The listing builds one solid part. Answer for the finished solid, in the listing's coordinates (mm). Give positions to 0.01 mm unless a question says otherwise; leave off trailing zeros. Order: outer loops, then holes, each group sorted by start corner. A loop starts at its lowest first (then second) coordinate and runs counter-clockwise, first axis right, second up. Notation, with made-up numbers: (76.25, 67.25) -> (105.25, 67.25) arc R34 cw to (105.25, 105.25) -> close; hole circle Ø3 at (32, 82). An arc over 180 degrees is marked (long way). One line per question, with ' | ' between items. Start each with the question number.
```python
from build123d import *

# Parameters (mm, degrees)
SKETCH1_R           = 28.194
BOSS_EXTRUDE1_DEPTH = 343
SKETCH5_R           = 28.194
BOSS_EXTRUDE3_DEPTH = 245
SKETCH7_R           = 3.675
CUT_EXTRUDE1_DEPTH  = 369.4


with BuildPart() as part:
    # Sketch1 → Boss-Extrude1 (new body)
    with BuildSketch(Plane(origin=(0, 0, 0), x_dir=(0, 0, -1), z_dir=(1, 0, 0))):
        Circle(SKETCH1_R)
    extrude(amount=BOSS_EXTRUDE1_DEPTH)

    # Sketch5 → Boss-Extrude3 (add)
    with BuildSketch(Plane(origin=(29.15, 29.15, 0), x_dir=(0.7071067811865464, -0.7071067811865488, 0), z_dir=(0.7071067811865488, 0.7071067811865464, 0))):
        with Locations(Location((41.224325343, 0, 0), (0, 0, 90))):
            Circle(SKETCH5_R)
    extrude(amount=BOSS_EXTRUDE3_DEPTH)

    # Sketch7 → Cut-Extrude1 (cut)
    with BuildSketch(Plane.ZY):
        Circle(SKETCH7_R)
    extrude(amount=-CUT_EXTRUDE1_DEPTH, mode=Mode.SUBTRACT)


solid = part.part
```
(1) The part is cut by section A-A on z = 0. Determine the outline of the cut face in (x, y) (3 decimals), plus the area to 3 significant figures.
(2) The part is cut by section C-C on x = 28. Determine the outline of the cut face in (y, z) (3 decimals), plus the area to 3 significant figures.
(3) The part is cut by section B-B on x = 196. State how many separate pieces and enclosed holes the cut face has, plus the area to 3 significant figures.
(4) Determine the mould class of faces 1 (the face through (231.26, 173.52, 0.39)), 2 (the face through (0, -6, 0)), 3 (the face through (169.099, -25.013, -13.01)) for opening direction Y: pulls with the +Y half, pulls with the -Y half, needs draft (parallel to the pull), parting line crosses it, or undercut.
(5) Consider line 1 (Y direction, x = 265, z = 0) (3 decimals); line 2 (Y direction, x = 171, z = 0) (3 decimals); line 3 (Y direction, x = 195, z = 0) (3 decimals). Determine where each line is inside the solid, lowest interval first.
(6) The part is cut by section D-D on z = -19. Determine the outline of the cut face in (x, y), plus the area to 3 significant figures.
(7) Given P1, Ø12, axis at x = 266, z = 2.5, coming from the +Y side; P2, Ø8, axis at y = 50, z = -16, coming from the +X side; P3, Ø5, axis at x = 207, y = 163, coming from the +Z side; P4, Ø6, axis at y = 0, z = 0, coming from the -X side, each flat-ended and moving along its own axis, determine where each tip first touches the part or whether it passes through.
Result sheet:
1) outline: (0, -28.194) -> (343, -28.194) -> (343, -3.675) -> (0, -3.675) -> close; (0, 3.675) -> (343, 3.675) -> (343, 28.194) -> (126.366, 28.194) -> (251.477, 153.305) -> (211.605, 193.177) -> (46.622, 28.194) -> (0, 28.194) -> close | area: 28,400 mm^2
2) outline: circle Ø56.388 at (0, 0); hole circle Ø7.35 at (0, 0) | area: 2,450 mm^2
3) separate pieces: 2 | enclosed holes: 1 | area: 5,990 mm^2
4) face 1: pulls with the +Y half | face 2: needs draft | face 3: undercut
5) line 1: y = -28.194 to -3.675, 3.675 to 28.194 | line 2: y = -28.194 to -3.675, 3.675 to 28.194, 72.828 to 152.572 | line 3: y = -28.194 to -3.675, 3.675 to 28.194, 96.828 to 176.572
6) outline: (0, -20.83) -> (343, -20.83) -> (343, 20.83) -> (108.59, 20.83) -> (246.27, 158.51) -> (216.81, 187.97) -> (49.67, 20.83) -> (0, 20.83) -> close | area: 23,300 mm^2
7) P1: stops at y = 28.19 | P2: stops at x = 146.43 | P3: stops at z = 27.15 | P4: passes through
